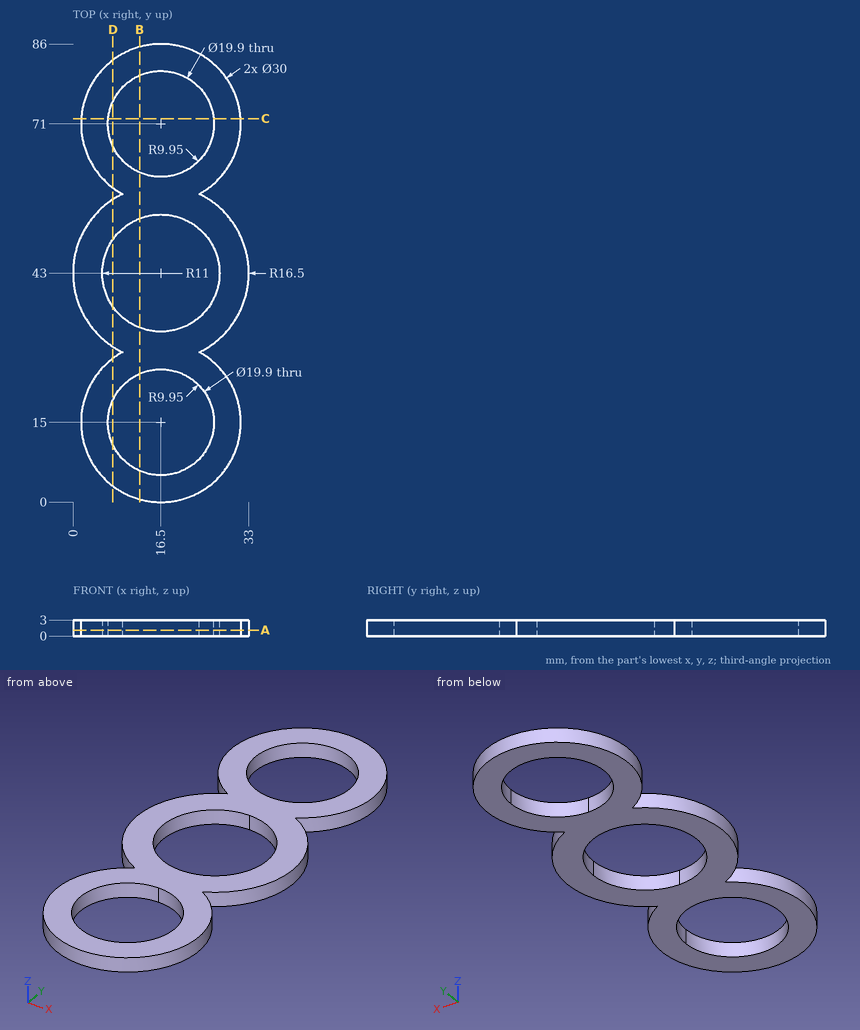
Design review of the part shown in the three views and the two pictorial views. Dimensions are in mm from the part's minimum x, y and z. Coordinates: 2 decimals unless noted, no trailing zeros. Order: outer loops, then holes, each group sorted by start corner. A loop starts at its lowest first (then second) coordinate and runs counter-clockwise, first axis right, second up. Notation, with made-up numbers: (-18.5, 1) - (33.5, 1) arc R6 cw to (33.5, 6) - close; hole circle Ø4 at (32.5, 30). An arc over 180 degrees is marked (long way). Answer as CSV lines item,"result". Start each with the question number.
1) Add section C-C (y = 72). State the section outline as (x, z) points, then the cut area to 3 significant figures.
2) Insertion check: P1, Ø12, axis at x = 16.5, y = 71, coming from the +Z side. The pin has a flat end and moves straight along its axis. Give the tip position at first contact, or say it passes through.
3) To check wall thickness, follow line 1 along Y through (x, z) = (16.5, 0.8); line 2 along Y through (x, z) = (6.5, 1.1); line 3 along X through (y, z) = (15, 1.1). State the ranges of each line that lie inside material, in increasing order. Write a range as [from, to].
4) Add section A-A (z = 1.15). State the section outline as (x, y) points, then the cut area to 3 significant figures.
5) Add section D-D (x = 7.5). State the section outline as (y, z) points.
6) Add section B-B (x = 12.5). State the section outline as (y, z) points.
Result:
1,outline,"(1.53, 0) - (6.6, 0) - (6.6, 3) - (1.53, 3) - close; (26.4, 0) - (31.47, 0) - (31.47, 3) - (26.4, 3) - close"
1,area,"30.4 mm^2"
2,P1,"through"
3,line 1,"[0, 5.05], [24.95, 32], [54, 61.05], [80.95, 86]"
3,line 2,"[3.82, 26.18], [29.88, 38.42], [47.58, 56.12], [59.82, 82.18]"
3,line 3,"[1.5, 6.55], [26.45, 31.5]"
4,outline,"(9.29, 28.16) arc R15 ccw (long way) to (23.71, 28.16) arc R16.5 ccw to (23.71, 57.84) arc R15 ccw (long way) to (9.29, 57.84) arc R16.5 ccw to start; hole (16.5, 24.95) arc R9.95 ccw (long way) to (26.45, 15) arc R9.95 ccw to start; hole (16.5, 32) arc R11 ccw to (27.5, 43) arc R11 ccw to (16.5, 54) arc R11 ccw to start; hole (16.5, 61.05) arc R9.95 ccw to (26.45, 71) arc R9.95 ccw (long way) to start"
4,area,"1,200 mm^2"
5,outline,"(3, 0) - (10.76, 0) - (10.76, 3) - (3, 3) - close; (19.24, 0) - (27, 0) - (27, 3) - (19.24, 3) - close; (29.17, 0) - (36.68, 0) - (36.68, 3) - (29.17, 3) - close; (49.32, 0) - (56.83, 0) - (56.83, 3) - (49.32, 3) - close; (59, 0) - (66.76, 0) - (66.76, 3) - (59, 3) - close; (75.24, 0) - (83, 0) - (83, 3) - (75.24, 3) - close"
6,outline,"(0.54, 0) - (5.89, 0) - (5.89, 3) - (0.54, 3) - close; (24.11, 0) - (32.75, 0) - (32.75, 3) - (24.11, 3) - close; (53.25, 0) - (61.89, 0) - (61.89, 3) - (53.25, 3) - close; (80.11, 0) - (85.46, 0) - (85.46, 3) - (80.11, 3) - close"
